```python
from build123d import *

# Parameters (mm, degrees)
SKETCH_1_R          = 5
SKETCH_1_R_2        = 2.5
EXTRUDE_1_DEPTH     = 8
SKETCH_2_R          = 5
SKETCH_2_R_2        = 4
CUT_EXTRUDE_1_DEPTH = 3


with BuildPart() as part:
    # 草图1 → 凸台-拉伸1 (new body)
    with BuildSketch(Plane(origin=(0, 0, 0), x_dir=(0, 0, -1), z_dir=(1, 0, 0))):
        Circle(SKETCH_1_R)
        Circle(SKETCH_1_R_2, mode=Mode.SUBTRACT)
    extrude(amount=EXTRUDE_1_DEPTH)

    # 草图2 → 切除-拉伸1 (cut, symmetric)
    with BuildSketch(Plane(origin=(4, 0, 0), x_dir=(0, 0, -1), z_dir=(1, 0, 0))):
        Circle(SKETCH_2_R)
        Circle(SKETCH_2_R_2, mode=Mode.SUBTRACT)
    extrude(amount=CUT_EXTRUDE_1_DEPTH, both=True, mode=Mode.SUBTRACT)


solid = part.part
```
Part model, mm, in its own coordinate system. Give positions to 0.01 mm unless a question says otherwise; leave off trailing zeros. Order: outer loops, then holes, each group sorted by start corner. A loop starts at its lowest first (then second) coordinate and runs counter-clockwise, first axis right, second up. Notation, with made-up numbers: M -17.75,70.5 L -8.75,70.5 A19 ccw -8.75,85.5 Z; hole C -11.5,67 d8. An arc over 180 degrees is marked long. Use a Markdown table: item, result. Add a question column.
(1) Saw through at A-A, the plane y = 0. Give the cut face in (x, z), and give its area (3 significant figures).
(2) Drop flat-ended pins along their axis: P1, Ø3, axis at x = 6, z = 1, coming from the +Y side; P2, Ø2, axis at x = 5.5, y = 2.5, coming from the -Z side; P3, Ø1.5, axis at x = 4, y = 0, coming from the -Z side; P4, Ø2, axis at x = 5, z = 1.5, coming from the -Y side. Give the stop position or say it passes through.
(3) Probe line 1 along Y through (x, z) = (3.25, 0); line 2 along X through (y, z) = (-0.5, 4); line 3 along Y through (x, z) = (0.5, 0). List the from-to ranges inside material, lowest first. Write a range as [from, to].
(4) Saw through at C-C, the plane x = 4.75. Give the cut face in (y, z), and give its area (3 significant figures).
(5) Mould opens along Y. For faces 1 (the face through (3.94, -2.44, 0.54)), 2 (the face through (8, -2, -2)), 3 (the face through (3.958, -3.905, 0.867)) say: +Y half, -Y half, draft (parallel to the pull), parting line (faces both ways), or undercut.
(6) Saw through at D-D, the plane z = -3. Give the cut face in (x, y).
Answer key:
| question | item | result |
|---|---|---|
| 1 | outline | M 0,-5 L 1,-5 L 1,-4 L 7,-4 L 7,-5 L 8,-5 L 8,-2.5 L 0,-2.5 Z; M 0,2.5 L 8,2.5 L 8,5 L 7,5 L 7,4 L 1,4 L 1,5 L 0,5 Z |
| 1 | area | 28.0 mm^2 |
| 2 | P1 | y = 5 |
| 2 | P2 | z = -3.71 |
| 2 | P3 | z = -4 |
| 2 | P4 | y = -3.97 |
| 3 | line 1 | [-4, -2.5], [2.5, 4] |
| 3 | line 2 | [0, 1], [7, 8] |
| 3 | line 3 | [-5, -2.5], [2.5, 5] |
| 4 | outline | C 0,0 d8; hole C 0,0 d5 |
| 4 | area | 30.6 mm^2 |
| 5 | face 1 | undercut |
| 5 | face 2 | draft |
| 5 | face 3 | parting line |
| 6 | outline | M 0,-4 L 1,-4 L 1,-2.65 L 7,-2.65 L 7,-4 L 8,-4 L 8,4 L 7,4 L 7,2.65 L 1,2.65 L 1,4 L 0,4 Z |
